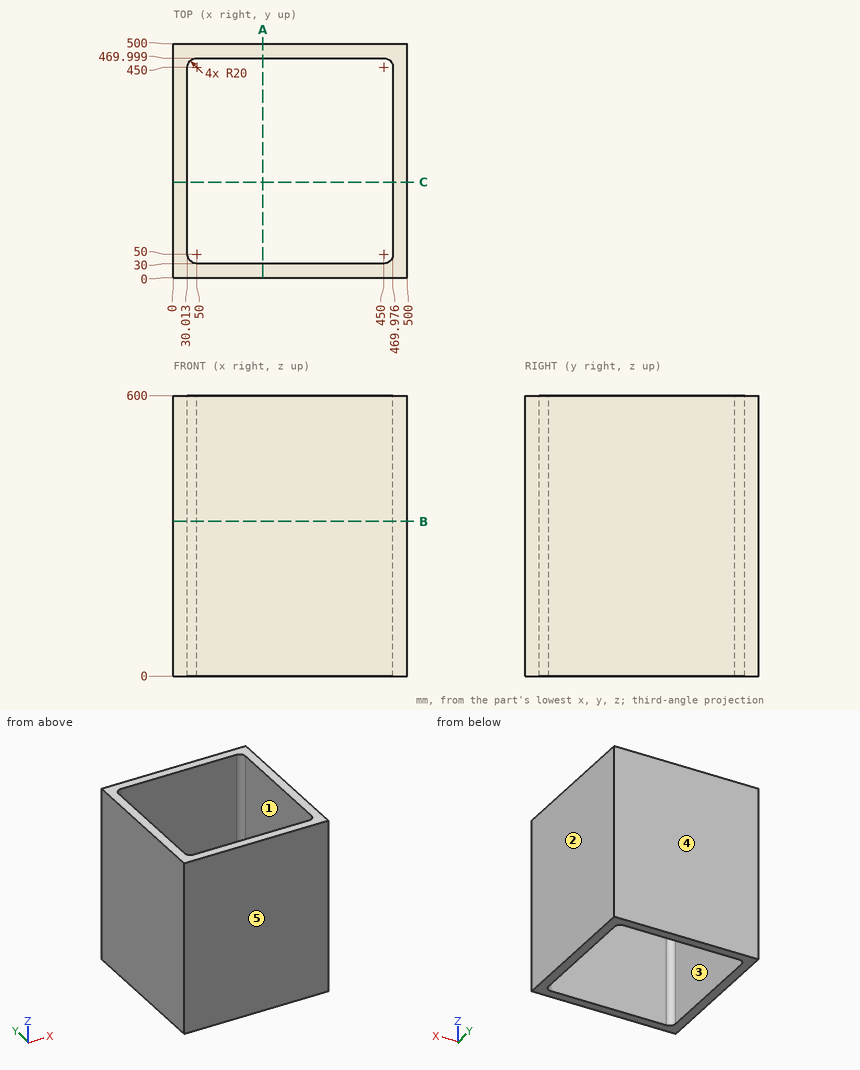
Design review of the part shown in the three views and the two pictorial views. Dimensions are in mm from the part's minimum x, y and z. A direction names the side the tool comes from. Give positions to 0.01 mm unless a question says otherwise; leave off trailing zeros. Loops run counter-clockwise (first coordinate to the right, second up) from the corner with the lowest first, then second, coordinate; pieces in that order, holes last. Notation, with made-up numbers: (-1, 68) -> (25, 68) arc R11 ccw to (25, 78) -> close; hole circle Ø9 at (65, 29). An arc over 180 degrees is marked (long way). Write each question's results on one line, items separated by ' | '.
Q1. Wall thickness on L1, parallel to Y at x = 256, z = 494; L2, parallel to X at y = 274, z = 414.5; L3, parallel to Y at x = 39, z = 277 (1 decimal): over which ranges is each line inside the solid? List them lowest first.
Reply:
L1: y = 0 to 30, 470 to 500 | L2: x = 0 to 30.01, 469.98 to 500 | L3: y = 0 to 33.3, 466.7 to 500
Q2. Take a section at B-B, the plane z = 331. Write out the cut boundary in (x, y) (1 decimal).
Reply:
outline: (0, 0) -> (500, 0) -> (500, 500) -> (0, 500) -> close; hole (30, 50.7) arc R20 ccw to (50.3, 30) -> (450, 30) arc R20 ccw to (470, 51) -> (470, 449) arc R20 ccw to (450, 470) -> (50.1, 470) arc R20 ccw to (30, 449.3) -> close
Q3. Take a section at C-C, the plane y = 204.5. Write out the cut boundary in (x, z), plus the area to 3 significant figures.
Reply:
outline: (0, 0) -> (30.01, 0) -> (30.01, 600) -> (0, 600) -> close; (469.98, 0) -> (500, 0) -> (500, 600) -> (469.98, 600) -> close | area: 36,000 mm²
Q4. Take a section at A-A, the plane x = 191.5. Write out the cut boundary in (y, z).
Reply:
outline: (0, 0) -> (30, 0) -> (30, 600) -> (0, 600) -> close; (470, 0) -> (500, 0) -> (500, 600) -> (470, 600) -> close
Q5. Machinability: for the marked faces 1 and 2, which of the approach directions +Z, -Z, +X, -X, +Y, -Y give a long, thin tool a straight path to every point of the face, cutting with its end or side? Answer none if there is none.
Reply:
face 1: +Z, -Z | face 2: +Z, -Z, +X, +Y, -Y
Q6. The part is to be moulded in two halves that separate along Y. For the marked faces 3, 4 and 5, say which applies: +Y half, -Y half, draft (parallel to the pull), parting line (faces both ways), or undercut.
Reply:
face 3: undercut | face 4: +Y half | face 5: -Y half
